Source: CAD feature listing. Evaluate the final solid. Frame: model axes, mm. A direction names the side the tool comes from. Give positions to 0.01 mm unless a question says otherwise; leave off trailing zeros. Write each loop counter-clockwise with the first axis right and the second up, starting at its lowest first coordinate (ties: lowest second). Pieces come first, ordered by that corner, then holes.
```python
from build123d import *

# Parameters (mm, degrees)
SKETCH5_R           = 1.4
BOSS_EXTRUDE1_DEPTH = 3


with BuildPart() as part:
    # Sketch5 → Boss-Extrude1 (new body)
    with BuildSketch(Plane(origin=(0, 0, 0), x_dir=(1, 0, 0), z_dir=(0, 1, 0))):
        with BuildLine():
            Line((-49.57228919, -87.412577044), (-62.57228919, -87.412577044))
            ThreePointArc((-62.57228919, -87.412577044), (0.15026567, 107.499894978), (62.32767078, -87.5871649))
            Line((62.32767078, -87.5871649), (49.32767078, -87.5871649))
            ThreePointArc((49.32767078, -87.5871649), (48.011633262, -81.999797234), (44.340215544, -77.5871649))
            Line((44.340215544, -77.5871649), (14.895351815, -60.5871649))
            Line((14.895351815, -60.5871649), (-15.104648185, -60.5871649))
            Line((-15.104648185, -60.5871649), (-44.549511914, -77.5871649))
            ThreePointArc((-44.549511914, -77.5871649), (-48.243794441, -81.895172415), (-49.57228919, -87.412577044))
        make_face()
        with Locations(Location((-93.103383397, 35.1, 0), (0, 0, 270))):
            Circle(SKETCH5_R, mode=Mode.SUBTRACT)
        with Locations(Location((35, 93.034187265, 0), (0, 0, 90))):
            Circle(SKETCH5_R, mode=Mode.SUBTRACT)
        with Locations(Location((-35, 93.034187265, 0), (0, 0, 270))):
            Circle(SKETCH5_R, mode=Mode.SUBTRACT)
        with Locations(Location((93.103383397, 35.1, 0), (0, 0, 90))):
            Circle(SKETCH5_R, mode=Mode.SUBTRACT)
        with Locations(Location((-11, -55.928525816, 0), (0, 0, 270))):
            Circle(SKETCH5_R, mode=Mode.SUBTRACT)
        with Locations(Location((11, -55.928525816, 0), (0, 0, 90))):
            Circle(SKETCH5_R, mode=Mode.SUBTRACT)
        with BuildLine():
            Line((-59.488560992, -64.166666667), (-20, -41.195529316))
            Line((-20, -41.195529316), (-20, 85.183625187))
            ThreePointArc((-20, 85.183625187), (-84.593056756, 22.366598952), (-59.488560992, -64.166666667))
        make_face(mode=Mode.SUBTRACT)
        with BuildLine():
            Line((-10, -40.5871649), (10, -40.5871649))
            Line((10, -40.5871649), (10, 86.926693254))
            ThreePointArc((10, 86.926693254), (0, 87.5), (-10, 86.926693254))
            Line((-10, 86.926693254), (-10, -40.5871649))
        make_face(mode=Mode.SUBTRACT)
        with BuildLine():
            Line((20, -41.195529316), (59.488560992, -64.166666667))
            ThreePointArc((59.488560992, -64.166666667), (84.593056756, 22.366598952), (20, 85.183625187))
            Line((20, 85.183625187), (20, -41.195529316))
        make_face(mode=Mode.SUBTRACT)
        Polygon((-100.9, -11.654989132), (-101.17241918, -8.667383437), (-91.17241918, -7.755552333), (-90.9, -10.743158028), align=None, mode=Mode.SUBTRACT)
        Polygon((-77.70280139, 66.108380167), (-75.71415707, 68.354553306), (-68.226913275, 61.725738906), (-70.215557595, 59.479565767), align=None, mode=Mode.SUBTRACT)
        Polygon((77.70280139, 66.108380167), (75.71415707, 68.354553306), (68.226913275, 61.725738906), (70.215557595, 59.479565767), align=None, mode=Mode.SUBTRACT)
        Polygon((100.9, -11.654989132), (90.9, -10.743158028), (91.17241918, -7.755552333), (101.17241918, -8.667383437), align=None, mode=Mode.SUBTRACT)
        Polygon((-61.179766354, -78.961014389), (-52.592640519, -73.836439294), (-51.055267991, -76.412577044), (-59.642393825, -81.537152139), align=None, mode=Mode.SUBTRACT)
        Polygon((52.592640519, -73.836439294), (51.055267991, -76.412577044), (59.642393825, -81.537152139), (61.179766354, -78.961014389), align=None, mode=Mode.SUBTRACT)
    extrude(amount=BOSS_EXTRUDE1_DEPTH)


solid = part.part
```
1. Cut plane D-D, the plane z = -24. Return the cut outline in (x, y).
2. Cut plane C-C, the plane x = -27. Return the cut outline in (y, z).
3. Line query: L1, parallel to X at y = 0.95, z = -1.5; L2, parallel to X at y = 0.9, z = -35.1; L3, parallel to Z at x = -77.5, y = 0.8. Output: solid intervals per line, ascending.
4. Contact query for flat-ended pins moving along their axis: P1, Ø1.7, axis at x = 11, z = 55.93, coming from the -Y side; P2, Ø0.9, axis at x = 2.5, y = 1.5, coming from the -Z side; P3, Ø1.5, axis at y = 2, z = 8.5, coming from the -X side; P4, Ø3, axis at x = -93.1, z = -35.1, coming from the +Y side. Output: stop coordinate, or through.
5. Cut plane A-A, the plane z = 0. Return the cut outline in (x, y), then the cut area to 3 significant figures.
6. Access query for faces 4 (the flat face through (-29.621, 1.479, 68.968)), 5 (the flat face through (-15, 3, -10)), 6 (the flat face through (56.946, 1.479, 76.435)). Directions: +Z, -Z, +X, -X, +Y, -Y. A direction counts if a zero-diameter tool reaches every point of the face in a straight line with its end or side. Return the directions, or none.
7. Cut plane B-B, the plane x = 0. Return the cut outline in (y, z), then the cut area to 3 significant figures.
8. Mould query, pull axis X, two halves, no side actions, for faces 1 (the flat face through (-15, 0, -10)), 2 (the cylindrical face through (-3.64, 1.48, -107.44)), 3 (the cylindrical face through (48.048, 1.479, 82.072)). Classes: +X half, -X half, draft (parallel to the pull), parting line (faces both ways), or undercut.
Response values:
1. outline: (-104.79, 0) - (-84.14, 0) - (-84.14, 3) - (-104.79, 3) - close; (-20, 0) - (-10, 0) - (-10, 3) - (-20, 3) - close; (10, 0) - (20, 0) - (20, 3) - (10, 3) - close; (84.14, 0) - (104.79, 0) - (104.79, 3) - (84.14, 3) - close
2. outline: (0, -104.05) - (3, -104.05) - (3, -83.23) - (0, -83.23) - close; (0, 45.27) - (3, 45.27) - (3, 67.45) - (0, 67.45) - close
3. L1: x = -107.49 to -87.49, -20 to -10, 10 to 20, 87.49 to 107.49
3. L2: x = -101.61 to -94.5, -91.7 to -80.15, -20 to -10, 10 to 20, 80.15 to 91.7, 94.5 to 101.61
3. L3: z = -74.5 to -66.34, -65.93 to -40.62, 40.62 to 74.5
4. P1: passes through
4. P2: stops at z = -107.48
4. P3: stops at x = -107.22
4. P4: stops at y = 3
5. outline: (-107.5, 0) - (-87.5, 0) - (-87.5, 3) - (-107.5, 3) - close; (-20, 0) - (-10, 0) - (-10, 3) - (-20, 3) - close; (10, 0) - (20, 0) - (20, 3) - (10, 3) - close; (87.5, 0) - (107.5, 0) - (107.5, 3) - (87.5, 3) - close
5. area: 180 mm2
6. face 4: +Z, +Y, -Y
6. face 5: +Z, -Z, +X, -X, +Y
6. face 6: +Y, -Y
7. outline: (0, -107.5) - (3, -107.5) - (3, -87.5) - (0, -87.5) - close; (0, 40.59) - (3, 40.59) - (3, 60.59) - (0, 60.59) - close
7. area: 120 mm2
8. face 1: draft
8. face 2: parting line
8. face 3: undercut
